The listing builds one solid part. Answer for the finished solid, in the listing's coordinates (mm). Give positions to 0.01 mm unless a question says otherwise; leave off trailing zeros. Write each loop counter-clockwise with the first axis right and the second up, starting at its lowest first coordinate (ties: lowest second). Pieces come first, ordered by that corner, then holes. Notation, with made-up numbers: M 49,49 L 82,49 A24 ccw 82,69 Z; hole C -1,39 d9. An arc over 180 degrees is marked long. Answer as a JSON object with one key per item and string values.
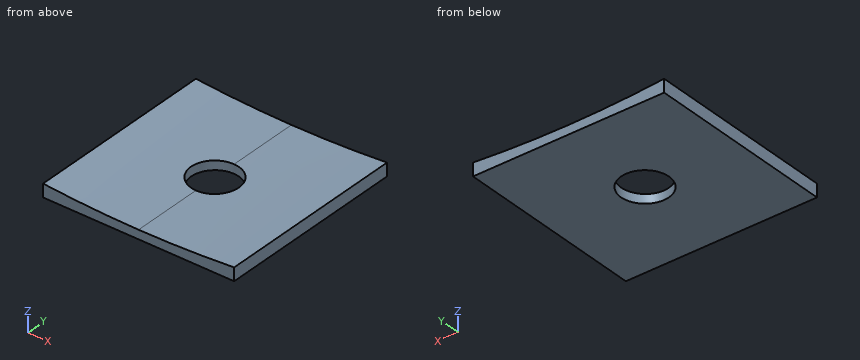
```python
from build123d import *

# Parameters (mm, degrees)
BOSS_EXTRUDE1_DEPTH = 25.4
SKETCH2_R           = 3.175
CUT_EXTRUDE1_DEPTH  = 1.7209262


with BuildPart() as part:
    # Sketch1 → Boss-Extrude1 (new body)
    with BuildSketch(Plane(origin=(0, 0, 0), x_dir=(1, 0, 0), z_dir=(0, 1, 0))):
        with BuildLine():
            Line((-12.7, 151.869911437), (-12.7, 153.590837637))
            Line((-12.7, 153.590837637), (12.7, 153.590837637))
            Line((12.7, 153.590837637), (12.7, 151.869911437))
            ThreePointArc((12.7, 151.869911437), (6.355528969, 152.267420191), (0, 152.4))
            ThreePointArc((0, 152.4), (-6.355528969, 152.267420191), (-12.7, 151.869911437))
        make_face()
    extrude(amount=-BOSS_EXTRUDE1_DEPTH)

    # Sketch2 → Cut-Extrude1 (cut)
    with BuildSketch(Plane(origin=(0, 0, -153.590837637), x_dir=(-1, 0, 0), z_dir=(0, 0, -1))):
        with Locations((0, -12.7)):
            Circle(SKETCH2_R)
    extrude(amount=-CUT_EXTRUDE1_DEPTH, mode=Mode.SUBTRACT)


solid = part.part
```
1. Flat-ended cylindrical pins translate along their axes: pin 1 (3 mm diameter, centred on x = 0, y = -10.5, fed in from +Z); pin 2 (6 mm diameter, centred on x = 8, y = -17, fed in from +Z). Find the tip coordinate at first contact, or state that the pin passes through.
Verdict:
{"pin 1": "stops at z = -152.39", "pin 2": "stops at z = -152"}
2. A cutting plane is placed at B-B, the plane x = 0.5. Give the vertices of the cut face in (y, z), plus the area to 3 significant figures.
Verdict:
{"outline": "M -25.4,-153.59 L -15.84,-153.59 L -15.84,-152.4 L -25.4,-152.4 Z; M -9.56,-153.59 L 0,-153.59 L 0,-152.4 L -9.56,-152.4 Z", "area": "22.8 mm2"}
3. A cutting plane is placed at A-A, the plane y = -12.7. Give the vertices of the cut face in (x, z) (3 decimals).
Verdict:
{"outline": "M -12.7,-153.591 L -3.175,-153.591 L -3.175,-152.367 A152.4 cw -12.7,-151.87 Z; M 3.175,-153.591 L 12.7,-153.591 L 12.7,-151.87 A152.4 cw 3.175,-152.367 Z"}
4. A cutting plane is placed at C-C, the plane y = -18.5. Give the vertices of the cut face in (x, z), plus the area to 3 significant figures.
Verdict:
{"outline": "M -12.7,-153.59 L 12.7,-153.59 L 12.7,-151.87 A152.4 cw -12.7,-151.87 Z", "area": "34.7 mm2"}
5. Consider line 1 along X through (y, z) = (-12.7, -152.65) (3 decimals); line 2 along Y through (x, z) = (0, -152.7) (3 decimals); line 3 along Z through (x, y) = (3, -6.25). Determine where each line is inside the solid, lowest interval first.
Verdict:
{"line 1": "x = -12.7 to -3.175, 3.175 to 12.7", "line 2": "y = -25.4 to -15.875, -9.525 to 0", "line 3": "z = -153.59 to -152.37"}
6. A cutting plane is placed at D-D, the plane x = -10. Give the vertices of the cut face in (y, z).
Verdict:
{"outline": "M -25.4,-153.59 L 0,-153.59 L 0,-152.07 L -25.4,-152.07 Z"}
